from build123d import *

# Parameters (mm, degrees)
F0_R             = 13.97
F1_DEPTH         = 3.175
F2_R             = 10.16
F3_DEPTH         = 2.1166666667
F4_R             = 10.16
F5_DEPTH         = 2.1166666667
F6_R             = 1.905
F7_DEPTH         = 2.54
F7_COPIES_COUNT  = 4
F8_R             = 3.81
F9_DEPTH         = 1.778
F10_R            = 3.81
F11_DEPTH        = 1.778
F13_DEPTH        = 6.35
F13_COPIES_COUNT = 30
F14_R            = 1.905
F15_DEPTH        = 5.6726666667


# Not quite as in the source:
# - a pattern or mirror of a feature is missing from the dataset's text; its kind, count and spacing are read off the source's solid


with BuildPart() as f1:
    # F0 (on Top) → F1 (new body, symmetric)
    with BuildSketch(Plane.XY):
        Circle(F0_R)
    extrude(amount=F1_DEPTH, both=True)

    # F2 (on face) → F3 (cut)
    with BuildSketch(Plane.XY.offset(3.175)):
        Circle(F2_R)
    extrude(amount=-F3_DEPTH, mode=Mode.SUBTRACT)

    # F4 (on face) → F5 (cut)
    with BuildSketch(Plane(origin=(0, 0, -3.175), x_dir=(1, 0, 0), z_dir=(0, 0, -1))):
        Circle(F4_R)
    extrude(amount=-F5_DEPTH, mode=Mode.SUBTRACT)

    # F6 (on face) → F7 (cut)
    with BuildSketch(Plane.XY.offset(1.0583333333)):
        with Locations((0, 6.985)):
            Circle(F6_R)
    f7 = extrude(amount=-F7_DEPTH, mode=Mode.SUBTRACT)

    # F7_copies: F7 ×4 about axis
    f7_copies_axis = Axis((0, 0, 0), (0, 0, 1))
    for i in range(1, F7_COPIES_COUNT):
        add(f7.rotate(f7_copies_axis, i * 360 / F7_COPIES_COUNT), mode=Mode.SUBTRACT)

    # F8 (on face) → F9 (join)
    with BuildSketch(Plane.XY.offset(1.0583333333)):
        Circle(F8_R)
    extrude(amount=F9_DEPTH)

    # F10 (on face) → F11 (join)
    with BuildSketch(Plane(origin=(0, 0, -1.0583333333), x_dir=(1, 0, 0), z_dir=(0, 0, -1))):
        Circle(F10_R)
    extrude(amount=F11_DEPTH)

    # F12 (on face) → F13 (join, through all)
    with BuildSketch(Plane.XY.offset(3.175)):
        Polygon((0, 17.0471984893), (-1.3763362913, 13.9020357651), (1.3763362913, 13.9020357651), align=None)
    f13 = extrude(amount=-F13_DEPTH)

    # F13_copies: F13 ×30 about axis
    f13_copies_axis = Axis((0, 0, 0), (0, 0, 1))
    for i in range(1, F13_COPIES_COUNT):
        add(f13.rotate(f13_copies_axis, i * 360 / F13_COPIES_COUNT))

    # F14 (on face) → F15 (cut, through all)
    with BuildSketch(Plane.XY.offset(2.8363333333)):
        Circle(F14_R)
    extrude(amount=-F15_DEPTH, mode=Mode.SUBTRACT)


solid = f1.part
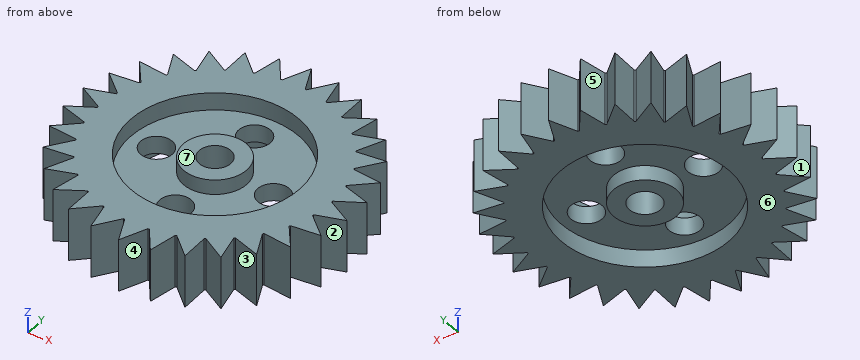
Build history of the part. All positions in model axes, mm. Face numbers are marked on the shaded views. A direction names the side the tool comes from. Round coordinates to 2 decimals unless told otherwise and drop trailing zeros. Loops run counter-clockwise (first coordinate to the right, second up) from the corner with the lowest first, then second, coordinate; pieces in that order, holes last. Notation, with made-up numbers: (29.5, 49) -> (44.5, 49) arc R21 cw to (44.5, 85) -> close; hole circle Ø2 at (-33.5, 46.25). An arc over 180 degrees is marked (long way). One line per item, written item: value. Start each with the question number.
Q1. Probe line 1 along Y through (x, z) = (12, -2.25); line 2 along Y through (x, z) = (0.5, -1.25); line 3 along Y through (x, z) = (15, 1.75). List the from-to ranges inside material, lowest first.
Q2. 3-axis set-ups, long thin cutter, end or side, ignore diameter. For the marked faces 1, 2, 3 and 4: which of +Z, -Z, +X, -X, +Y, -Y reach the whole face in a straight line?
Q3. Two-plate mould, pull along Y, no slides. Class the marked faces 5, 6 and 7: released by +Y, released by -Y, zero draft, split by the parting line, or undercut.
Q4. Cut at A-A on z = 1.5. Count the separate pieces of the cut face and the enclosed holes in it, plus the area to 3 significant figures.
Q5. Drop flat-ended pins along their axis: pin 1 Ø1 at (x, z) = (-12, 2.5) entering from -Y; pin 2 Ø5 at (x, y) = (6.985, 0) entering from -Z; pin 3 Ø12 at (x, y) = (0, 0) entering from +Z. Give the stop position or say it passes through.
Q6. Cut at B-B on y = 15. List the corners of the cut face in (x, z) (3 decimals).
Computed:
1. line 1: -11.18 to -9.93, -8.22 to 8.22, 9.93 to 11.18
1. line 2: -15.9 to -10.15, -3.78 to -1.84, 1.84 to 3.78, 10.15 to 15.9
1. line 3: -5.39 to -4.19, -2.4 to -0.67, 0.67 to 2.4, 4.19 to 5.39
2. face 1: +Z, -Z, -X
2. face 2: +Z, -Z, +X
2. face 3: +Z, -Z
2. face 4: +Z, -Z, -Y
3. face 5: released by +Y
3. face 6: zero draft
3. face 7: undercut
4. separate pieces: 2
4. enclosed holes: 2
4. area: 449 mm²
5. pin 1: y = -11.35
5. pin 2: z = -1.06
5. pin 3: z = 2.84
6. outline: (-6.93, -3.175) -> (-6.305, -3.175) -> (-6.305, 3.175) -> (-6.93, 3.175) -> close; (-3.889, -3.175) -> (-2.344, -3.175) -> (-2.344, 3.175) -> (-3.889, 3.175) -> close; (-0.896, -3.175) -> (0.896, -3.175) -> (0.896, 3.175) -> (-0.896, 3.175) -> close; (2.344, -3.175) -> (3.889, -3.175) -> (3.889, 3.175) -> (2.344, 3.175) -> close; (6.305, -3.175) -> (6.93, -3.175) -> (6.93, 3.175) -> (6.305, 3.175) -> close
